Here's how the part is built. I have some questions about the finished solid (model axes, mm). Round coordinates to 2 decimals unless told otherwise and drop trailing zeros. Write each loop counter-clockwise with the first axis right and the second up, starting at its lowest first coordinate (ties: lowest second). Pieces come first, ordered by that corner, then holes. Notation, with made-up numbers: (9.25, 62) -> (65.25, 62) arc R25 cw to (65.25, 84) -> close; hole circle Ø2 at (5, 54.5). An arc over 180 degrees is marked (long way). Answer in a Markdown table with one row per item. Add a question column.
from build123d import *

# Parameters (mm, degrees)
SKETCH1_W                = 69.85
SKETCH1_H                = 100.5
BOSS_EXTRUDE1_DEPTH      = 7
FILLET1_R                = 3
M3_CLEARANCE_HOLE1_D     = 3.4
M3_CLEARANCE_HOLE1_DEPTH = 2
M3_CLEARANCE_HOLE1_TIP   = 1.021463052
M3_CLEARANCE_HOLE2_D     = 3.4
SKETCH6_W                = 39.454447737
SKETCH6_H                = 3.466414688
CUT_EXTRUDE1_DEPTH       = 5


with BuildPart() as part:
    # Sketch1 → Boss-Extrude1 (new body)
    with BuildSketch(Plane.XY):
        with Locations((34.925, 50.25)):
            Rectangle(SKETCH1_W, SKETCH1_H)
    extrude(amount=BOSS_EXTRUDE1_DEPTH)

    # Fillet1
    fillet1_edges = [part.edges().sort_by_distance(p)[0] for p in [
        (0, 100.5, 3.5),
        (69.85, 100.5, 3.5),
        (69.85, 0, 3.5),
        (0, 0, 3.5),
    ]]
    fillet(fillet1_edges, radius=FILLET1_R)

    # M3 Clearance Hole1
    with Locations(Plane(origin=(4.07, 86.5, 0), x_dir=(-1, 0, 0), z_dir=(0, 0, -1))):
        with Locations((0, 0), (-61.71, 0), (-61.71, -76.6), (0, -76.6)):
            Hole(M3_CLEARANCE_HOLE1_D / 2, depth=M3_CLEARANCE_HOLE1_DEPTH)
            with Locations((0, 0, -(M3_CLEARANCE_HOLE1_DEPTH + M3_CLEARANCE_HOLE1_TIP / 2))):  # 118° drill point
                Cone(0, M3_CLEARANCE_HOLE1_D / 2, M3_CLEARANCE_HOLE1_TIP, mode=Mode.SUBTRACT)

    # M3 Clearance Hole2 (through all)
    with Locations(Plane(origin=(0, 86.5, 3), x_dir=(0, 0, -1), z_dir=(-1, 0, 0))):
        with Locations((0, 0), (0, 76.6)):
            Hole(M3_CLEARANCE_HOLE2_D / 2)

    # Sketch6 → Cut-Extrude1 (cut)
    with BuildSketch(Plane(origin=(0, 100.5, 0), x_dir=(1, 0, 0), z_dir=(0, 1, 0))):
        with Locations((33.611063607, -1.733207344)):
            Rectangle(SKETCH6_W, SKETCH6_H)
    extrude(amount=-CUT_EXTRUDE1_DEPTH, mode=Mode.SUBTRACT)


solid = part.part
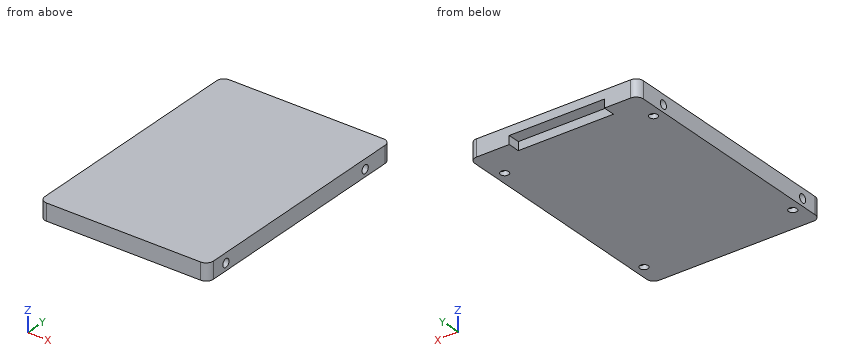
Item 1: If we section it at B-B on y = 86.5: Please give me the cut outline in (x, z), then the cut area to 3 significant figures.
Item 2: If we section it at C-C on x = 60.5: Please give me the cut outline in (y, z).
Item 3: I need wall thicknesses on line 1 along Y through (x, z) = (65.78, 0.4); line 2 along Y through (x, z) = (53.5, 2); line 3 along Z through (x, y) = (34.5, 9). Which ranges of each line are inside material? Lowest first, please. Write a range as from..to.
Item 4: If we section it at A-A on x = 45.5: Please give me the cut outline in (y, z), then the cut area to 3 significant figures.
Item 5: For P1, Ø3, axis at x = 43, z = 1, coming from the +Y side; P2, Ø2, axis at x = 4.07, y = 86.5, coming from the -Z side; P3, Ø2, axis at y = 86.5, z = 3, coming from the -X side; P4, Ø2.5, axis at x = 29.5, y = 97, coming from the -Z side, each with a flat end and sliding along its axis, tell me the tip position at first contact or that it passes through.
Results list:
| question | item | result |
|---|---|---|
| 1 | outline | (0, 0) -> (2.37, 0) -> (2.37, 1.3) -> (0, 1.3) -> close; (0, 4.7) -> (69.85, 4.7) -> (69.85, 7) -> (0, 7) -> close; (5.77, 0) -> (64.08, 0) -> (64.08, 1.3) -> (5.77, 1.3) -> close; (67.48, 0) -> (69.85, 0) -> (69.85, 1.3) -> (67.48, 1.3) -> close |
| 1 | area | 243 mm² |
| 2 | outline | (0, 0) -> (100.5, 0) -> (100.5, 7) -> (0, 7) -> close; hole circle Ø3.4 at (9.9, 3); hole circle Ø3.4 at (86.5, 3) |
| 3 | line 1 | 0..8.2, 11.6..84.8, 88.2..100.5 |
| 3 | line 2 | 0..8.53, 11.27..85.13, 87.87..100.5 |
| 3 | line 3 | 0..1.56, 4.44..7 |
| 4 | outline | (0, 0) -> (95.5, 0) -> (95.5, 3.47) -> (100.5, 3.47) -> (100.5, 7) -> (0, 7) -> close; hole circle Ø3.4 at (9.9, 3); hole circle Ø3.4 at (86.5, 3) |
| 4 | area | 668 mm² |
| 5 | P1 | y = 95.5 |
| 5 | P2 | z = 4.37 |
| 5 | P3 | through |
| 5 | P4 | z = 3.47 |
